Could you check a few things on this model? Use its own coordinates, in mm. Coordinates: 2 decimals unless noted, no trailing zeros. Loops run counter-clockwise (first coordinate to the right, second up) from the corner with the lowest first, then second, coordinate; pieces in that order, holes last. Notation, with made-up numbers: (-34, 1) - (-30, 1) arc R17 cw to (-30, 26) - close; hole circle Ø8 at (-40, -13.5). An arc over 180 degrees is marked (long way). One line per item, written item: value. Start each with the question number.
(1) If I drill on line 1 along Y through (x, z) = (6.5, 5); line 2 along Y through (x, z) = (5.5, 4); line 3 along Y through (x, z) = (6.5, -9.5), over which ranges is the centre line in solid material (lowest first)? Write a range as from..to.
(2) If we section it at B-B on x = 6.5: Write out the boundary of the cut face in (y, z), then the cut area to 3 significant figures.
(3) I'm going to push flat-ended pins straight in: P1, Ø10, axis at y = -30.5, z = -13.5, coming from the +X side; P2, Ø3, axis at x = 6.5, y = -2.9, coming from the -Z side. Where does each tip first touch, or does it pass through?
(4) If we section it at A-A on z = -13.5: Write out the boundary of the cut face in (x, y), then the cut area to 3 significant figures.
(5) If we section it at D-D on x = 2.75: Write out the boundary of the cut face in (y, z).
(6) If we section it at C-C on z = -9: Write out the boundary of the cut face in (x, y), then the cut area to 3 significant figures.
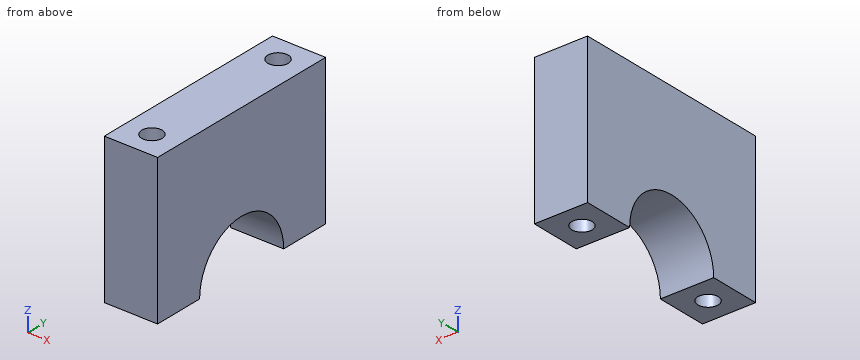
```python
from build123d import *

# Parameters (mm, degrees)
F1_DEPTH = 13
F2_R     = 2.5
F4_DEPTH = 36
F3_R     = 2.5
F5_DEPTH = 36


with BuildPart() as f1:
    # F0 (on Right) → F1 (new body)
    with BuildSketch(Plane.YZ):
        with BuildLine():
            Line((3.351025, 17.020911), (-46.648975, 17.020911))
            Line((-46.648975, 17.020911), (-46.648975, -18.979089))
            Line((-46.648975, -18.979089), (-34.148975, -18.979089))
            ThreePointArc((-34.148975, -18.979089), (-21.648975, -6.479089), (-9.148975, -18.979089))
            Line((-9.148975, -18.979089), (3.351025, -18.979089))
            Line((3.351025, -18.979089), (3.351025, 17.020911))
        make_face()
    extrude(amount=F1_DEPTH)

    # F2 (on face) → F4 (cut)
    with BuildSketch(Plane(origin=(0, 0, -18.979089), x_dir=(1, 0, 0), z_dir=(0, 0, -1))):
        with Locations((6.5, 40.398975)):
            Circle(F2_R)
    extrude(amount=-F4_DEPTH, mode=Mode.SUBTRACT)

    # F3 (on face) → F5 (cut)
    with BuildSketch(Plane(origin=(0, 0, -18.979089), x_dir=(1, 0, 0), z_dir=(0, 0, -1))):
        with Locations((6.5, 2.898975)):
            Circle(F3_R)
    extrude(amount=-F5_DEPTH, mode=Mode.SUBTRACT)


solid = f1.part
```
Values:
1. line 1: y = -46.65..-42.9, -37.9..-5.4, -0.4..3.35
1. line 2: y = -46.65..-42.69, -38.11..-5.19, -0.61..3.35
1. line 3: y = -46.65..-42.9, -37.9..-29.8, -13.5..-5.4, -0.4..3.35
2. outline: (-46.65, -18.98) - (-42.9, -18.98) - (-42.9, 17.02) - (-46.65, 17.02) - close; (-37.9, -18.98) - (-34.15, -18.98) arc R12.5 cw to (-9.15, -18.98) - (-5.4, -18.98) - (-5.4, 17.02) - (-37.9, 17.02) - close; (-0.4, -18.98) - (3.35, -18.98) - (3.35, 17.02) - (-0.4, 17.02) - close
2. area: 1,190 mm2
3. P1: stops at x = 13
3. P2: passes through
4. outline: (0, -46.65) - (13, -46.65) - (13, -32.88) - (0, -32.88) - close; (0, -10.41) - (13, -10.41) - (13, 3.35) - (0, 3.35) - close; hole circle Ø5 at (6.5, -40.4); hole circle Ø5 at (6.5, -2.9)
4. area: 319 mm2
5. outline: (-46.65, -18.98) - (-34.15, -18.98) arc R12.5 cw to (-9.15, -18.98) - (3.35, -18.98) - (3.35, 17.02) - (-46.65, 17.02) - close
6. outline: (0, -46.65) - (13, -46.65) - (13, -29.18) - (0, -29.18) - close; (0, -14.12) - (13, -14.12) - (13, 3.35) - (0, 3.35) - close; hole circle Ø5 at (6.5, -40.4); hole circle Ø5 at (6.5, -2.9)
6. area: 415 mm2
